Design review of the part built by this model. Coordinates are the model's own, in mm. Round coordinates to 2 decimals unless told otherwise and drop trailing zeros. Loops run counter-clockwise (first coordinate to the right, second up) from the corner with the lowest first, then second, coordinate; pieces in that order, holes last. Notation, with made-up numbers: (59, -22.75) -> (67, -22.75) arc R19 ccw to (67, -10.75) -> close; hole circle Ø1 at (35.25, 88.25). An arc over 180 degrees is marked (long way). Answer as CSV lines item,"result". Start each with the question number.
```python
from build123d import *

# Parameters (mm, degrees)
SKETCH_1_R      = 0.4
EXTRUDE_1_DEPTH = 10
SKETCH_2_W      = 90
SKETCH_2_H      = 0.8
EXTRUDE_2_DEPTH = 0.8
FILLET_1_R      = 0.4
SKETCH_3_R      = 0.4
EXTRUDE_3_DEPTH = 5
SKETCH_4_R      = 0.4
EXTRUDE_4_DEPTH = 5
CHAMFER_1_SIZE  = 0.4


with BuildPart() as part:
    # 草图1 → 凸台-拉伸1 (new body)
    with BuildSketch(Plane(origin=(0, 0, 0), x_dir=(1, 0, 0), z_dir=(0, 1, 0))):
        with Locations(Location((0, 0, 0), (0, 0, 270))):
            Circle(SKETCH_1_R)
    extrude(amount=EXTRUDE_1_DEPTH)

    # 草图2 → 凸台-拉伸2 (add)
    with BuildSketch(Plane(origin=(0, 10, 0), x_dir=(1, 0, 0), z_dir=(0, 1, 0))):
        Rectangle(SKETCH_2_W, SKETCH_2_H)
    extrude(amount=EXTRUDE_2_DEPTH)

    # 圆角1
    fillet_1_edges = [part.edges().sort_by_distance(p)[0] for p in [
        (45, 10, 0),
        (45, 10.8, 0),
        (-45, 10, 0),
        (-45, 10.8, 0),
    ]]
    fillet(fillet_1_edges, radius=FILLET_1_R - 0.0001)  # a hair under: the kernel refuses the full size

    # 草图3 → 凸台-拉伸3 (add)
    with BuildSketch(Plane.XY.offset(0.4)):
        with Locations((44.6, 10.4)):
            Circle(SKETCH_3_R)
    extrude(amount=EXTRUDE_3_DEPTH)

    # 草图4 → 凸台-拉伸4 (add)
    with BuildSketch(Plane(origin=(0, 0, -0.4), x_dir=(-1, 0, 0), z_dir=(0, 0, -1))):
        with Locations((44.6, 10.4)):
            Circle(SKETCH_4_R)
    extrude(amount=EXTRUDE_4_DEPTH)

    # 倒角1
    chamfer_1_edges = [part.edges().sort_by_distance(p)[0] for p in [
        (44.2, 10.4, 5.4),
        (-44.2, 10.4, -5.4),
    ]]
    chamfer(chamfer_1_edges, length=CHAMFER_1_SIZE)


solid = part.part
```
Q1. Add section C-C, the plane z = -2.25. Give the boundary of the cut face in (x, y).
Q2. To check wall thickness, follow probe 1 along X at (y, z) = (3, 0); probe 2 along X at (y, z) = (10.25, -4.5). State the ranges of each line that lie inside material, in increasing order. Write a range as from..to.
Q3. Add section B-B, the plane y = 7. Give the boundary of the cut face in (x, z), and give its area (3 significant figures).
Q4. Add section A-A, the plane x = -37.5. Give the boundary of the cut face in (y, z).
Q5. For pin 1 Ø0.6 at (x, y) = (7.5, 10.5) entering from +Z; pin 2 Ø5 at (y, z) = (9.5, 3.5) entering from -X; pin 3 Ø1.5 at (y, z) = (8.5, 4.5) entering from -X; pin 4 Ø0.6 at (x, z) = (-17.5, 0) entering from -Y, all flat-tipped, find the tip position at first contact; note any pin that passes through.
Worked answers:
1,outline,"circle Ø0.8 at (-44.6, 10.4)"
2,probe 1,"x = -0.4..0.4"
2,probe 2,"x = -44.97..-44.23"
3,outline,"circle Ø0.8 at (0, 0)"
3,area,"0.503 mm^2"
4,outline,"(10, -0.4) -> (10.8, -0.4) -> (10.8, 0.4) -> (10, 0.4) -> close"
5,pin 1,"stops at z = 0.4"
5,pin 2,"stops at x = 44.2"
5,pin 3,"passes through"
5,pin 4,"stops at y = 10"
